Geometry: final body of the model. Coordinates: model frame, mm. A direction names the side the tool comes from. Give positions to 0.01 mm unless a question says otherwise; leave off trailing zeros. Write each loop counter-clockwise with the first axis right and the second up, starting at its lowest first coordinate (ties: lowest second). Pieces come first, ordered by that corner, then holes. Notation, with made-up numbers: (15, 8) -> (63, 8) arc R22 cw to (63, 14) -> close; hole circle Ø4 at (40, 16). An arc over 180 degrees is marked (long way). Answer in a Markdown table with one row per item. Add a question column.
Item 1: Material intervals for probe 1 along X at (y, z) = (-10, 8); probe 2 along Y at (x, z) = (13, 4.5); probe 3 along Y at (x, z) = (35, 3.5), sorted ascending. Write a range as from..to.
Item 2: Section query D-D on x = 39.5. Output: boundary loops of the cut face in (y, z).
Item 3: Section query C-C on x = -10.5. Output: boundary loops of the cut face in (y, z).
Item 4: Access query for faces 1 (the flat face through (-13.456, 0, 5)), 2 (the flat face through (0, 16, 0)). Directions: +Z, -Z, +X, -X, +Y, -Y. A direction counts if a zero-diameter tool reaches every point of the face in a straight line with its end or side. Return the directions, or none.
Item 5: Section query B-B on z = 6.75. Output: boundary loops of the cut face in (x, y).
Item 6: Section query A-A on y = 14. Output: boundary loops of the cut face in (x, z).
Item 7: First-contact query: P1, Ø3, axis at x = 18.5, z = 2.5, coming from the -Y side; P2, Ø5, axis at y = -2.5, z = 7, coming from the +X side. Flat tips, straight axial feed; report the tip coordinate or a pass-through.
```python
from build123d import *

# Parameters (mm, degrees)
F0_W     = 6
F0_H     = 50
F1_DEPTH = 10


with BuildPart() as f1:
    # F0 (on Top) → F1 (new body)
    with BuildSketch(Plane.XY):
        Polygon((-19.455582, 33.734061), (-19.455582, 25.734061), (-13.455582, 25.734061), (-5.455582, 25.734061), (0.544418, 25.734061), (30.544418, 25.734061), (50.544418, 18.734061), (50.544418, 33.734061), align=None)
        with Locations((-16.455582, 0.734061)):
            Rectangle(F0_W, F0_H)
        with Locations((-2.455582, 0.734061)):
            Rectangle(F0_W, F0_H)
    extrude(amount=F1_DEPTH)


with BuildPart() as f2_1:
    # F2: copy of F1
    add(f1.part)


solid = f1.part
```
Findings below:
| question | item | result |
|---|---|---|
| 1 | probe 1 | x = -19.46..-13.46, -5.46..0.54 |
| 1 | probe 2 | y = 25.73..33.73 |
| 1 | probe 3 | y = 24.17..33.73 |
| 2 | outline | (22.6, 0) -> (33.73, 0) -> (33.73, 10) -> (22.6, 10) -> close |
| 3 | outline | (25.73, 0) -> (33.73, 0) -> (33.73, 10) -> (25.73, 10) -> close |
| 4 | face 1 | +Z, -Z, -Y |
| 4 | face 2 | -Z, +X, -X, +Y, -Y |
| 5 | outline | (-19.46, -24.27) -> (-13.46, -24.27) -> (-13.46, 25.73) -> (-5.46, 25.73) -> (-5.46, -24.27) -> (0.54, -24.27) -> (0.54, 25.73) -> (30.54, 25.73) -> (50.54, 18.73) -> (50.54, 33.73) -> (-19.46, 33.73) -> close |
| 6 | outline | (-19.46, 0) -> (-13.46, 0) -> (-13.46, 10) -> (-19.46, 10) -> close; (-5.46, 0) -> (0.54, 0) -> (0.54, 10) -> (-5.46, 10) -> close |
| 7 | P1 | stops at y = 25.73 |
| 7 | P2 | stops at x = 0.54 |
